```python
from build123d import *

# Parameters (mm, degrees)
BASE_SHAPE_DEPTH    = 17
SKETCH4_W           = 10
SKETCH4_H           = 13.5
WING_CUT_OUTS_DEPTH = 16.5
SKETCH5_R           = 1.75
WING_HOLES_DEPTH    = 119.380741677
SKETCH7_W           = 14
SKETCH7_H           = 14
CUT_EXTRUDE1_DEPTH  = 114.5
SKETCH8_W           = 14
SKETCH8_H           = 14
CUT_EXTRUDE2_DEPTH  = 25.5
CUT_EXTRUDE3_DEPTH  = 14
SKETCH10_R          = 2.6
CUT_EXTRUDE4_DEPTH  = 121.307938225


with BuildPart() as part:
    # Sketch1 → Base Shape (new body)
    with BuildSketch(Plane.XY):
        with BuildLine():
            Line((0, 18.313708499), (0, 94))
            Line((0, 94), (-5, 99))
            Line((-5, 99), (-10, 99))
            Line((-10, 99), (-10, 116))
            Line((-10, 116), (17, 116))
            Line((17, 116), (17, 18.313708499))
            ThreePointArc((17, 18.313708499), (17.60896374, 15.25224104), (19.343145751, 12.656854249))
            Line((19.343145751, 12.656854249), (27, 5))
            Line((27, 5), (27, 0))
            Line((27, 0), (17, 0))
            Line((17, 0), (0, 0))
            Line((0, 0), (-10, 0))
            Line((-10, 0), (-10, 5))
            Line((-10, 5), (-2.343145751, 12.656854249))
            ThreePointArc((-2.343145751, 12.656854249), (-0.60896374, 15.25224104), (0, 18.313708499))
        make_face()
    extrude(amount=BASE_SHAPE_DEPTH)

    # Sketch4 → Wing Cut Outs (cut)
    with BuildSketch(Plane(origin=(0, 2, 0), x_dir=(-1, 0, 0), z_dir=(0, -1, 0))):
        with Locations((5, -8)):
            Rectangle(SKETCH4_W, SKETCH4_H)
    wing_cut_outs = extrude(amount=-WING_CUT_OUTS_DEPTH, mode=Mode.SUBTRACT)

    # Sketch5 → Wing Holes (cut, through all)
    with BuildSketch(Plane(origin=(0, 2, 0), x_dir=(-1, 0, 0), z_dir=(0, -1, 0))):
        with Locations(Location((5, -8, 0), (0, 0, 180))):
            Circle(SKETCH5_R)
    wing_holes = extrude(amount=WING_HOLES_DEPTH, mode=Mode.SUBTRACT)

    # Mirror1: Wing Cut Outs across plane
    add(wing_cut_outs.mirror(Plane(origin=(8.5, 0, 0), x_dir=(0, 0, 1), z_dir=(1, 0, 0))), mode=Mode.SUBTRACT)

    # Mirror2: Wing Holes across plane
    add(wing_holes.mirror(Plane(origin=(8.5, 0, 0), x_dir=(0, 0, 1), z_dir=(1, 0, 0))), mode=Mode.SUBTRACT)

    # Sketch7 → Cut-Extrude1 (cut)
    with BuildSketch(Plane(origin=(0, 0, 0), x_dir=(1, 0, 0), z_dir=(0, 1, 0))):
        with Locations((8.5, -8.5)):
            Rectangle(SKETCH7_W, SKETCH7_H)
    extrude(amount=CUT_EXTRUDE1_DEPTH, mode=Mode.SUBTRACT)

    # Sketch8 → Cut-Extrude2 (cut)
    with BuildSketch(Plane(origin=(-10, 0, 0), x_dir=(0, 0, -1), z_dir=(1, 0, 0))):
        with Locations((-8.5, 107.5)):
            Rectangle(SKETCH8_W, SKETCH8_H)
    extrude(amount=CUT_EXTRUDE2_DEPTH, mode=Mode.SUBTRACT)

    # Sketch9 → Cut-Extrude3 (cut)
    with BuildSketch(Plane.XY.offset(1.5)):
        Polygon((1.5, 94.621320344), (-4.378679656, 100.5), (1.5, 100.5), align=None)
    extrude(amount=CUT_EXTRUDE3_DEPTH, mode=Mode.SUBTRACT)

    # Sketch10 → Cut-Extrude4 (cut, through all)
    with BuildSketch(Plane.XY):
        with Locations((10.5, 107.5)):
            Circle(SKETCH10_R)
        with Locations((-4.5, 107.5)):
            Circle(SKETCH10_R)
    extrude(amount=CUT_EXTRUDE4_DEPTH, mode=Mode.SUBTRACT)


solid = part.part
```
Work out the finished part from the listing and answer in its coordinate system (mm). A direction names the side the tool comes from. Give positions to 0.01 mm unless a question says otherwise; leave off trailing zeros. Order: outer loops, then holes, each group sorted by start corner. A loop starts at its lowest first (then second) coordinate and runs counter-clockwise, first axis right, second up. Notation, with made-up numbers: (31, 27.25) - (47, 27.25) arc R19 ccw to (47, 38.25) - close; hole circle Ø4 at (79, 2). An arc over 180 degrees is marked (long way). One line per item, written item: value. Start each with the question number.
1. For a pull along Z with two mould halves and no side action, classify faces 1 (the face through (23.75, 1.01, 8.08)), 2 (the face through (-0.626, 15.212, 15.859)) as released by +Z, released by -Z, zero draft, split by the parting line, or undercut.
2. Each of these flat-tipped pins is pushed along its axis until it touches: pin 1 Ø7 at (y, z) = (33, 6.5) entering from -X; pin 2 Ø4 at (x, z) = (20, 9) entering from +Y; pin 3 Ø8.5 at (y, z) = (33, 7) entering from +X. Where does it stop, or does it pass through?
3. Section C-C, the plane y = 80 is taken. Write down the section's boundary in (x, z).
4. Which of the six approach directions +Z, -Z, +X, -X, +Y, -Y give full straight-line access (tool end or side, diameter ignored) to faces 3 (the face through (-4, 6, 14.75)), 4 (the face through (-5.228, 1.014, 9.735)), 5 (the face through (-7, 99, 8)), 6 (the face through (21, 6, 14.75)), 7 (the face through (-1.4, 97.52, 8.4))?
5. Section D-D, the plane x = 10.5 is taken. Write down the section's boundary in (y, z), then the cut area to 3 significant figures.
6. Section B-B, the plane x = 22 is taken. Write down the section's boundary in (y, z), then the cut area to 3 significant figures.
7. Consider line 1 (X direction, y = 107.5, z = 16); line 2 (Y direction, x = -5, z = 13.25); line 3 (Z direction, x = 9, y = 103.5). Determine where each line is inside the solid, lowest interval first.
8. Section A-A, the plane z = 8 is taken. Write down the section's boundary in (x, y).
Filled sheet:
1. face 1: undercut
1. face 2: zero draft
2. pin 1: x = 0
2. pin 2: y = 2
2. pin 3: x = 17
3. outline: (0, 0) - (17, 0) - (17, 17) - (0, 17) - close; hole (1.5, 1.5) - (15.5, 1.5) - (15.5, 15.5) - (1.5, 15.5) - close
4. face 3: -X
4. face 4: -Y
4. face 5: +Z, -Z, -X
4. face 6: +X, +Y
4. face 7: none
5. outline: (0, 0) - (104.9, 0) - (104.9, 1.5) - (0, 1.5) - close; (0, 15.5) - (104.9, 15.5) - (104.9, 17) - (0, 17) - close; (110.1, 0) - (116, 0) - (116, 17) - (110.1, 17) - (110.1, 15.5) - (114.5, 15.5) - (114.5, 1.5) - (110.1, 1.5) - close
5. area: 353 mm²
6. outline: (0, 0) - (10, 0) - (10, 1.25) - (2, 1.25) - (2, 6.25) - (0, 6.25) - close; (0, 9.75) - (2, 9.75) - (2, 14.75) - (10, 14.75) - (10, 17) - (0, 17) - close
6. area: 55.0 mm²
7. line 1: -10 to -7.1, -1.9 to 7.9, 13.1 to 17
7. line 2: 0 to 2, 99 to 100.5, 114.5 to 116
7. line 3: 0 to 1.5, 15.5 to 17
8. outline: (-10, 0) - (-6.75, 0) - (-6.75, 2) - (-10, 2) - close; (-10, 99) - (-5, 99) - (0, 94) - (0, 2) - (-3.25, 2) - (-3.25, 0) - (1.5, 0) - (1.5, 94.62) - (-4.38, 100.5) - (-10, 100.5) - close; (-10, 114.5) - (15.5, 114.5) - (15.5, 0) - (20.25, 0) - (20.25, 2) - (17, 2) - (17, 116) - (-10, 116) - close; (23.75, 0) - (27, 0) - (27, 2) - (23.75, 2) - close
